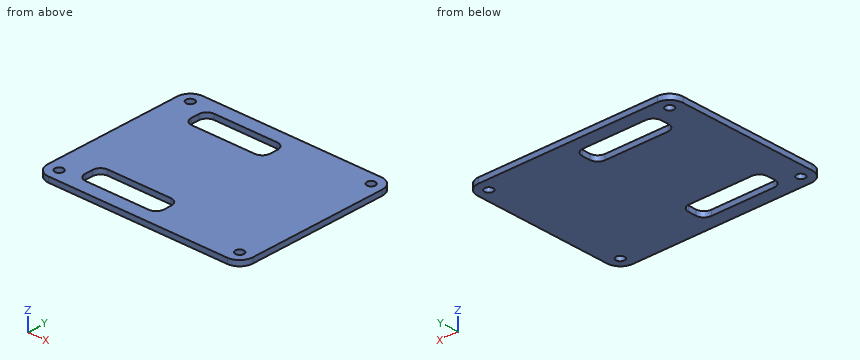
Autodesk Inventor part; units mm, degrees
ref_plane "YZ Plane" through (0, 0, 0) normal (1, 0, 0) x (0, 1, 0)
ref_plane "XZ Plane" through (0, 0, 0) normal (0, 1, 0) x (-1, 0, 0)
ref_plane "XY Plane" through (0, 0, 0) normal (0, 0, 1) x (1, 0, 0)
sketch "Kort" plane through (0, 0, 0) normal (0, 0, 1) x (1, 0, 0)
  line L0 (-3.0921, 63.9853) -> (22.7279, 63.9853)
  line L1 (22.7279, 63.9853) -> (22.7279, 58.9853)
  line L2 (22.7279, 58.9853) -> (-3.0921, 58.9853)
  line L3 (-3.0921, 58.9853) -> (-3.0921, 63.9853)
  line L4 (-2.9921, 20.7153) -> (22.8179, 20.7153)
  line L5 (22.8179, 20.7153) -> (22.8179, 15.7153)
  line L6 (22.8179, 15.7153) -> (-2.9921, 15.7153)
  line L7 (-2.9921, 15.7153) -> (-2.9921, 20.7153)
  line L8 (-14.2921, 69.1953) -> (59.3579, 69.1953)
  line L9 (-14.2921, 10.6153) -> (-14.2921, 69.1953)
  line L10 (59.3579, 10.6153) -> (-14.2921, 10.6153)
  line L11 (59.3579, 69.1953) -> (59.3579, 10.6153)
  circle A0 centre (56.8329, 66.5703) radius 1.575
  circle A1 centre (56.7329, 13.2403) radius 1.575
  circle A2 centre (-11.6671, 66.5703) radius 1.575
  circle A3 centre (-11.6671, 13.2403) radius 1.575
  line L12 (61.3579, 71.1953) -> (-16.2921, 71.1953)
  line L13 (-16.2921, 71.1953) -> (-16.2921, 8.6153)
  line L14 (-16.2921, 8.6153) -> (61.3579, 8.6153)
  line L15 (61.3579, 8.6153) -> (61.3579, 71.1953)
  line L16 (24.7279, 65.9853) -> (-5.0921, 65.9853)
  line L17 (-5.0921, 65.9853) -> (-5.0921, 56.9853)
  line L18 (-5.0921, 56.9853) -> (24.7279, 56.9853)
  line L19 (24.7279, 56.9853) -> (24.7279, 65.9853)
  line L20 (24.8179, 22.7153) -> (-4.9921, 22.7153)
  line L21 (-4.9921, 22.7153) -> (-4.9921, 13.7153)
  line L22 (-4.9921, 13.7153) -> (24.8179, 13.7153)
  line L23 (24.8179, 13.7153) -> (24.8179, 22.7153)
  point P0 (0, 0)
  dimension "d4" = 5.21
  dimension "d5" = 11.2
  dimension "d6" = 5.1
  dimension "d7" = 11.3
  dimension "d8" = 5
  dimension "d9" = 5
  dimension "d10" = 25.82
  dimension "d11" = 25.81
  dimension "d12" = 58.58
  dimension "d13" = 73.65
  dimension "d14" = 2.625
  dimension "d15" = 2.525
  dimension "d16" = 3.15
  dimension "d17" = 3.15
  dimension "d18" = 3.15
  dimension "d19" = 3.15
  dimension "d20" = 2.625
  dimension "d21" = 2.625
  dimension "d22" = 2.625
  dimension "d23" = 2.625
  dimension "d24" = 2.625
  dimension "d25" = 2.625
  dimension "d26" = 2
  dimension "d27" = 2
  dimension "d28" = 2
extrude "Bottom" add sketch "Kort" along normal blind 2 contours L8 L11 L10 L9 | L15 L14 L13 L12
fillet "Kantutjevning" radius 5 4 edges at (61.3579, 8.6153, 1) (61.3579, 71.1953, 1) (-16.2921, 71.1953, 1) (-16.2921, 8.6153, 1)
fillet "Hullkantutjevning" radius 3 8 edges at (-5.0921, 65.9853, 1) (-5.0921, 56.9853, 1) (24.7279, 65.9853, 1) (24.8179, 22.7153, 1) (24.7279, 56.9853, 1) (24.8179, 13.7153, 1) (-4.9921, 13.7153, 1) (-4.9921, 22.7153, 1)
equation "\"BendRadius\" = Thickness"
equation "\"BendReliefWidth\" = Thickness"
equation "\"BendReliefDepth\" = 0.5 * Thickness"
equation "\"CornerReliefSize\" = 4 * Thickness"
equation "\"MinimumRemnant\" = 2 * Thickness"
equation "\"TransitionRadius\" = BendRadius"
equation "\"JacobiRadiusSize\" = BendRadius"
equation "\"GapSize\" = Thickness"
properties part number "Trippeldekker_Nedre plate"
Source: CAD feature listing. Evaluate the final solid. Frame: model axes, mm. Coordinates: 2 decimals unless noted, no trailing zeros. Loops run counter-clockwise (first coordinate to the right, second up) from the corner with the lowest first, then second, coordinate; pieces in that order, holes last. Notation, with made-up numbers: (78, 46.5) -> (113, 46.5) arc R30 cw to (113, 71.5) -> close; hole circle Ø6 at (83.25, 34.5). An arc over 180 degrees is marked (long way). One line per item, written item: value. Start each with the question number.
Q1. Line query: line 1 along Y through (x, z) = (0, 1.45); line 2 along Y through (x, z) = (58, 0.4); line 3 along X through (y, z) = (60.5, 1.25). Output: solid intervals per line, ascending.
Q2. Section query A-A, the plane x = 5. Return the cut outline in (y, z), and give its area (3 significant figures).
Q3. Section query B-B, the plane z = 1.6. Return the cut outline in (x, y) (3 decimals).
Results:
1. line 1: 8.62 to 13.72, 22.72 to 56.99, 65.99 to 71.2
1. line 2: 8.89 to 12.3, 14.18 to 65.51, 67.63 to 70.92
1. line 3: -16.29 to -5.09, 24.73 to 61.36
2. outline: (8.62, 0) -> (13.72, 0) -> (13.72, 2) -> (8.62, 2) -> close; (22.72, 0) -> (56.99, 0) -> (56.99, 2) -> (22.72, 2) -> close; (65.99, 0) -> (71.2, 0) -> (71.2, 2) -> (65.99, 2) -> close
2. area: 89.2 mm^2
3. outline: (-16.292, 13.615) arc R5 ccw to (-11.292, 8.615) -> (56.358, 8.615) arc R5 ccw to (61.358, 13.615) -> (61.358, 66.195) arc R5 ccw to (56.358, 71.195) -> (-11.292, 71.195) arc R5 ccw to (-16.292, 66.195) -> close; hole circle Ø3.15 at (-11.667, 13.24); hole circle Ø3.15 at (-11.667, 66.57); hole (-5.092, 59.985) arc R3 ccw to (-2.092, 56.985) -> (21.728, 56.985) arc R3 ccw to (24.728, 59.985) -> (24.728, 62.985) arc R3 ccw to (21.728, 65.985) -> (-2.092, 65.985) arc R3 ccw to (-5.092, 62.985) -> close; hole (-4.992, 16.715) arc R3 ccw to (-1.992, 13.715) -> (21.818, 13.715) arc R3 ccw to (24.818, 16.715) -> (24.818, 19.715) arc R3 ccw to (21.818, 22.715) -> (-1.992, 22.715) arc R3 ccw to (-4.992, 19.715) -> close; hole circle Ø3.15 at (56.733, 13.24); hole circle Ø3.15 at (56.833, 66.57)
